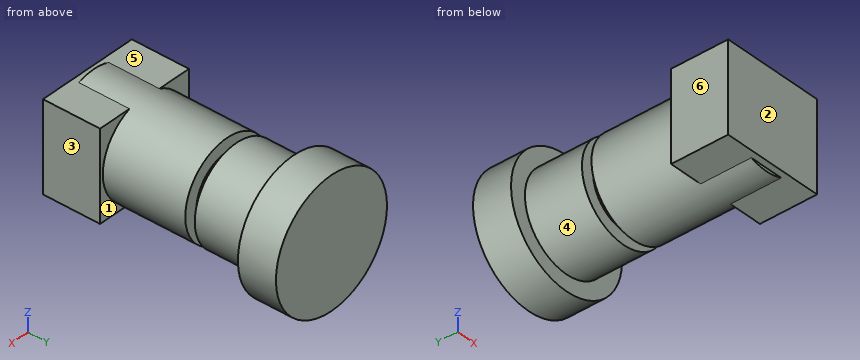
```python
from build123d import *

# Parameters (mm, degrees)
SK_P02_CONTACTBLOCKSNC1NC2_W  = 32
SK_P02_CONTACTBLOCKSNC1NC2_H  = 28
P02_CONTACTBLOCKSNC1NC2_DEPTH = 18


with BuildPart() as part:
    # SK_P01_Mushroomandbody → P01_Mushroomandbody (revolve)
    with BuildSketch(Plane.XY, mode=Mode.PRIVATE) as p01_mushroomandbody_sk:
        Polygon((0, 2), (15, 2), (15, 44), (11, 44), (11, 47), (15, 47), (15, 65), (20, 65), (20, 77), (0, 77), align=None)
    revolve(p01_mushroomandbody_sk.sketch.rotate(Axis((0, -3, 0), (0, 1, 0)), 90), axis=Axis((0, -3, 0), (0, 1, 0)))

    # SK_P02_ContactblocksNC1NC2 → P02_ContactblocksNC1NC2 (add)
    with BuildSketch(Plane(origin=(0, 0, 0), x_dir=(1, 0, 0), z_dir=(0, 1, 0))):
        Rectangle(SK_P02_CONTACTBLOCKSNC1NC2_W, SK_P02_CONTACTBLOCKSNC1NC2_H)
    extrude(amount=P02_CONTACTBLOCKSNC1NC2_DEPTH)


solid = part.part
```
Design review of the part built by this model. Coordinates are the model's own, in mm. Face numbers are marked on the shaded views. A direction names the side the tool comes from. Coordinates: 2 decimals unless noted, no trailing zeros. Order: outer loops, then holes, each group sorted by start corner. A loop starts at its lowest first (then second) coordinate and runs counter-clockwise, first axis right, second up.
1) Wall thickness on line 1 along Y through (x, z) = (-11, -12); line 2 along Y through (x, z) = (1, 12); line 3 along Z through (x, y) = (6, 4): over which ranges is each line inside the solid? List them lowest first.
2) Take a section at D-D, the plane y = 22. Give the boundary of the cut face in (x, z), and give its area (3 significant figures).
3) For the marked faces 4, 5 and 6, list the 3-axis set-ups (+Z, -Z, +X, -X, +Y, -Y) from which the entire face can be reached by the end or side of a thin tool; tool diameter is ignored.
4) Mouldability with a two-part tool opening along Y and no side actions: class the marked faces 1, 2 and 3 as +Y half, -Y half, draft (parallel to the pull), parting line (faces both ways), or undercut.
5) Clearance check with flat-ended pins moving along their axes: pin 1 (10 mm diameter, centred on y = 34.5, z = -16, fed in from +X); pin 2 (20 mm diameter, centred on x = 9, z = 8.5, fed in from -Y); pin 3 (9 mm diameter, centred on x = 6, y = 7.5, fed in from -Z); pin 4 (3 mm diameter, centred on y = 61.5, z = -10.5, fed in from +X). State where each tip first meets the part, or that it passes through.
6) Take a section at B-B, the plane y = 12. Give the boundary of the cut face in (x, z).
7) Take a section at C-C, the plane z = -8. Give the boundary of the cut face in (x, y).
8) Take a section at A-A, the plane x = 0. Give the boundary of the cut face in (y, z).
Returned:
1. line 1: y = 0 to 18, 65 to 77
1. line 2: y = 0 to 44, 47 to 77
1. line 3: z = -14 to 14
2. outline: circle Ø30 at (0, 0)
2. area: 707 mm2
3. face 4: none
3. face 5: +Z, -Y
3. face 6: +Z, -Z, -X, -Y
4. face 1: undercut
4. face 2: -Y half
4. face 3: draft
5. pin 1: stops at x = 10.2
5. pin 2: stops at y = 0
5. pin 3: stops at z = -14.92
5. pin 4: stops at x = 12
6. outline: (-16, -14) - (-5.39, -14) arc R15 ccw to (5.39, -14) - (16, -14) - (16, 14) - (5.39, 14) arc R15 ccw to (-5.39, 14) - (-16, 14) - close
7. outline: (-18.33, 65) - (-12.69, 65) - (-12.69, 47) - (-7.55, 47) - (-7.55, 44) - (-12.69, 44) - (-12.69, 18) - (-16, 18) - (-16, 0) - (16, 0) - (16, 18) - (12.69, 18) - (12.69, 44) - (7.55, 44) - (7.55, 47) - (12.69, 47) - (12.69, 65) - (18.33, 65) - (18.33, 77) - (-18.33, 77) - close
8. outline: (0, -14) - (2, -14) - (2, -15) - (44, -15) - (44, -11) - (47, -11) - (47, -15) - (65, -15) - (65, -20) - (77, -20) - (77, 20) - (65, 20) - (65, 15) - (47, 15) - (47, 11) - (44, 11) - (44, 15) - (2, 15) - (2, 14) - (0, 14) - close
